from build123d import *

# Parameters (mm, degrees)
SKETCH1_W           = 11.176
SKETCH1_H           = 25.4
BOSS_EXTRUDE1_DEPTH = 6.35
SKETCH2_R           = 3.302
CUT_EXTRUDE1_DEPTH  = 7.874
CUT_EXTRUDE2_REACH  = 17.259
SKETCH3_R           = 1.63195


with BuildPart() as part:
    # Sketch1 → Boss-Extrude1 (new body)
    with BuildSketch(Plane(origin=(0, 0, 0), x_dir=(1, 0, 0), z_dir=(0, 1, 0))):
        Rectangle(SKETCH1_W, SKETCH1_H)
    extrude(amount=-BOSS_EXTRUDE1_DEPTH)

    # Sketch2 → Cut-Extrude1 (cut)
    with BuildSketch(Plane.ZY.offset(5.588)):
        Circle(SKETCH2_R)
    extrude(amount=-CUT_EXTRUDE1_DEPTH, mode=Mode.SUBTRACT)

    # Sketch3 → Cut-Extrude2 (cut, up to next)
    with BuildSketch(Plane(origin=(0, 0, 0), x_dir=(1, 0, 0), z_dir=(0, 1, 0)), mode=Mode.PRIVATE) as cut_extrude2_sk1:
        with Locations(Location((0, 7.874, 0), (0, 0, 270))):
            Circle(SKETCH3_R)
    cut_extrude2_tool1 = extrude(cut_extrude2_sk1.sketch, amount=-CUT_EXTRUDE2_REACH, mode=Mode.PRIVATE) & part.part
    # Sketch3 → Cut-Extrude2 (cut, up to next)
    with BuildSketch(Plane(origin=(0, 0, 0), x_dir=(1, 0, 0), z_dir=(0, 1, 0)), mode=Mode.PRIVATE) as cut_extrude2_sk2:
        with Locations(Location((0, -7.874, 0), (0, 0, 270))):
            Circle(SKETCH3_R)
    cut_extrude2_tool2 = extrude(cut_extrude2_sk2.sketch, amount=-CUT_EXTRUDE2_REACH, mode=Mode.PRIVATE) & part.part
    add(cut_extrude2_tool1.solids().sort_by_distance((0, 0, -7.874))[0], mode=Mode.SUBTRACT)
    add(cut_extrude2_tool2.solids().sort_by_distance((0, 0, 7.874))[0], mode=Mode.SUBTRACT)


solid = part.part
The listing builds one solid part. Answer for the finished solid, in the listing's coordinates (mm). A direction names the side the tool comes from. Coordinates: 2 decimals unless noted, no trailing zeros. Order: outer loops, then holes, each group sorted by start corner. A loop starts at its lowest first (then second) coordinate and runs counter-clockwise, first axis right, second up. Notation, with made-up numbers: M 24,3.5 L 55,3.5 A20 cw 55,14.5 Z; hole C -9,31.5 d8. An arc over 180 degrees is marked long. Use CSV: the item, a comma, the result in double quotes.
Q1. Section B-B (z = 8) is taken. Determine the outline of the cut face in (x, y), then the cut area to 3 significant figures.
Here are the results:
outline,"M -5.59,-6.35 L -1.63,-6.35 L -1.63,0 L -5.59,0 Z; M 1.63,-6.35 L 5.59,-6.35 L 5.59,0 L 1.63,0 Z"
area,"50.3 mm2"
Q2. Section D-D (x = -2) is taken. Determine the outline of the cut face in (y, z).
Here are the results:
outline,"M -6.35,-12.7 L 0,-12.7 L 0,-3.3 A3.3 cw 0,3.3 L 0,12.7 L -6.35,12.7 Z"
Q3. A tool of negligible diameter and unlimited length cuts with its end or side. For faces 1 (the flat face through (4, 0, 0)), 2 (the flat face through (2.286, -1, 0)), from which of +Z, -Z, +X, -X, +Y, -Y can it reach the whole face along a straight path? Write none if from no direction.
Here are the results:
face 1,"+Z, -Z, +X, -X, +Y"
face 2,"-X, +Y"
Q4. Section C-C (y = -0.75) is taken. Determine the outline of the cut face in (x, z).
Here are the results:
outline,"M -5.59,-12.7 L 5.59,-12.7 L 5.59,12.7 L -5.59,12.7 L -5.59,3.22 L 2.29,3.22 L 2.29,-3.22 L -5.59,-3.22 Z; hole C 0,-7.87 d3.26; hole C 0,7.87 d3.26"
Q5. Section A-A (x = 0) is taken. Determine the outline of the cut face in (y, z), then the cut area to 3 significant figures.
Here are the results:
outline,"M -6.35,-12.7 L 0,-12.7 L 0,-9.51 L -6.35,-9.51 Z; M -6.35,-6.24 L 0,-6.24 L 0,-3.3 A3.3 cw 0,3.3 L 0,6.24 L -6.35,6.24 Z; M -6.35,9.51 L 0,9.51 L 0,12.7 L -6.35,12.7 Z"
area,"103 mm2"
Q6. Straight lines are drawn through the part: L1, parallel to Z at x = -0.25, y = -5.75; L2, parallel to X at y = -2, z = -1.25; L3, parallel to X at y = -5.5, z = 9.25. For each, find the intervals that lie inside material, in ascending order.
Here are the results:
L1,"-12.7 to -9.49, -6.26 to 6.26, 9.49 to 12.7"
L2,"2.29 to 5.59"
L3,"-5.59 to -0.88, 0.88 to 5.59"
Q7. Given pin 1 Ø1 at (y, z) = (-1.5, -0.5) entering from -X; pin 2 Ø6 at (x, z) = (-2, -1) entering from +Y; pin 3 Ø2.5 at (x, z) = (0, 7.874) entering from +Y, each flat-ended and moving along its own axis, determine where each tip first touches the part or whether it passes through.
Here are the results:
pin 1,"x = 2.29"
pin 2,"y = 0"
pin 3,"through"
Q8. Determine the mould class of faces 3 (the cylindrical face through (0.072, -3.131, -9.504)), 4 (the flat face through (-5.588, -4, 0)), 5 (the flat face through (0, -6.35, 0)) for opening direction X: pulls with the +X half, pulls with the -X half, needs draft (parallel to the pull), parting line crosses it, or undercut.
Here are the results:
face 3,"undercut"
face 4,"pulls with the -X half"
face 5,"needs draft"
